Verification items for this drawing (mm, ordinates from the low corner). Round coordinates to 2 decimals unless told otherwise and drop trailing zeros. Order: outer loops, then holes, each group sorted by start corner. A loop starts at its lowest first (then second) coordinate and runs counter-clockwise, first axis right, second up. Notation, with made-up numbers: (-29, 63) -> (10, 63) arc R18 ccw to (10, 71) -> close; hole circle Ø6 at (22.5, 67.5). An arc over 180 degrees is marked (long way). Use a Markdown table: item, result. Add a question column.
Item 1: Sectioned sample at A-A, the plane y = 7. Record the cut outline in (x, z).
Item 2: Sectioned sample at C-C, the plane x = 22. Record the cut outline in (y, z), and give its area (3 significant figures).
Item 3: Gauge pin test, flat ends, axial feed: pin 1 Ø1 at (x, z) = (3, 1) entering from +Y; pin 2 Ø1 at (x, z) = (7, 1) entering from -Y; pin 3 Ø1.5 at (x, z) = (15, 3) entering from -Y. Record the tip position at first contact, or that the pin passes through.
Item 4: Mould release check, pull along Y, two halves, no side actions. Record for the marked faces 1, 2, 3 and 4: pulls with the +Y half, pulls with the -Y half, needs draft (parallel to the pull), parting line crosses it, or undercut.
Item 5: Sectioned sample at D-D, the plane z = 4.25. Record the cut outline in (x, y), and give its area (3 significant figures).
Item 6: Material ranges on probe 1 along Y at (x, z) = (15.75, 8); probe 2 along Y at (x, z) = (10.75, 6.2); probe 3 along X at (y, z) = (7.25, 10.75), recorded low to high. Write a range as [from, to].
Item 7: Sectioned sample at B-B, the plane x = 16.5. Record the cut outline in (y, z), and give its area (3 significant figures).
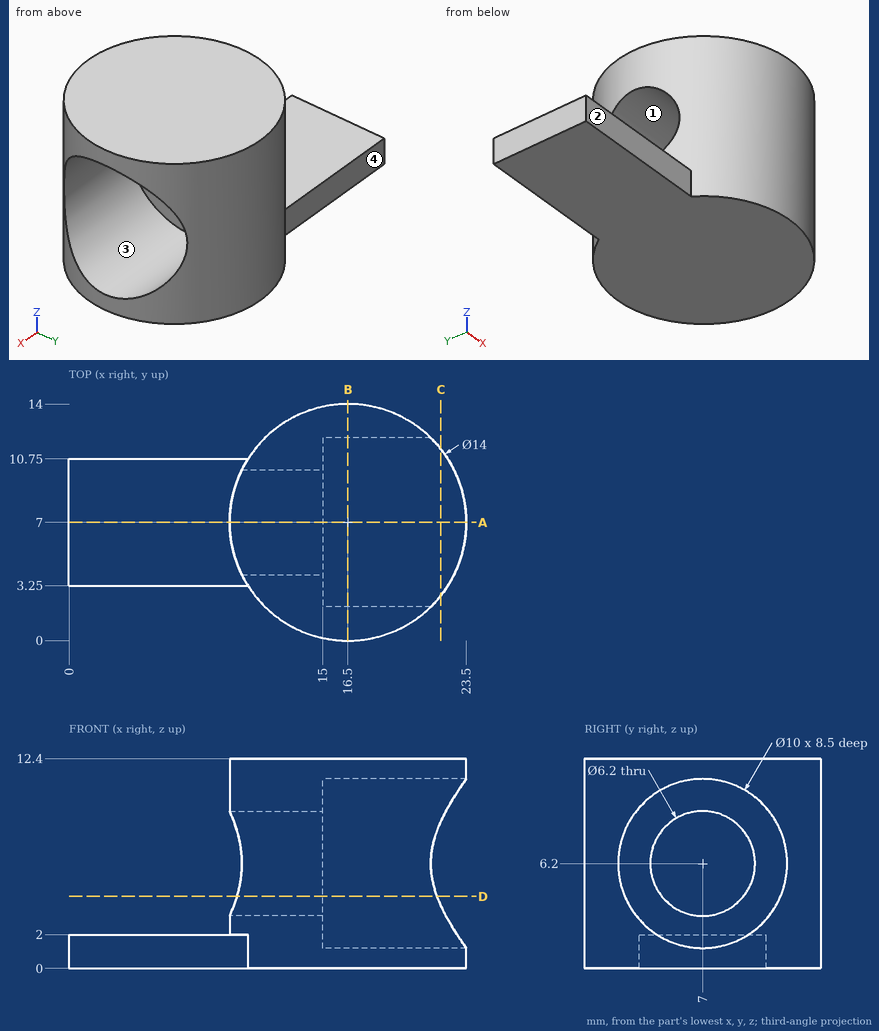
Found:
| question | item | result |
|---|---|---|
| 1 | outline | (0, 0) -> (23.5, 0) -> (23.5, 1.2) -> (15, 1.2) -> (15, 3.1) -> (9.5, 3.1) -> (9.5, 2) -> (0, 2) -> close; (9.5, 9.3) -> (15, 9.3) -> (15, 11.2) -> (23.5, 11.2) -> (23.5, 12.4) -> (9.5, 12.4) -> close |
| 2 | outline | (2.67, 0) -> (11.33, 0) -> (11.33, 3.7) arc R5 cw to (2.67, 3.7) -> close; (2.67, 8.7) arc R5 cw to (11.33, 8.7) -> (11.33, 12.4) -> (2.67, 12.4) -> close |
| 2 | area | 33.4 mm2 |
| 3 | pin 1 | stops at y = 10.75 |
| 3 | pin 2 | stops at y = 3.25 |
| 3 | pin 3 | stops at y = 0.04 |
| 4 | face 1 | undercut |
| 4 | face 2 | pulls with the -Y half |
| 4 | face 3 | undercut |
| 4 | face 4 | pulls with the +Y half |
| 5 | outline | (9.93, 4.59) arc R7 ccw to (21.77, 2.4) -> (15, 2.4) -> (15, 4.59) -> close; (9.93, 9.41) -> (15, 9.41) -> (15, 11.6) -> (21.77, 11.6) arc R7 ccw to start |
| 5 | area | 54.8 mm2 |
| 6 | probe 1 | y = [0.04, 2.34], [11.66, 13.96] |
| 6 | probe 2 | y = [3.01, 3.9], [10.1, 10.99] |
| 6 | probe 3 | x = [9.5, 15] |
| 7 | outline | (0, 0) -> (14, 0) -> (14, 12.4) -> (0, 12.4) -> close; hole circle Ø10 at (7, 6.2) |
| 7 | area | 95.1 mm2 |
